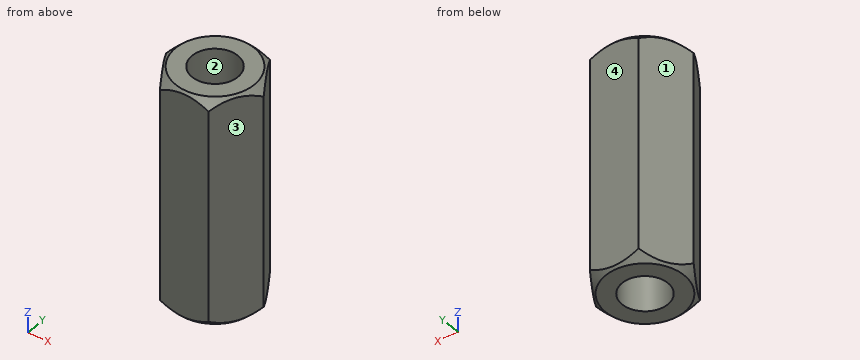
```python
from build123d import *

# Parameters (mm, degrees)
EXTRUDE_1_DEPTH   = 4
HOLE_WIZARD_M21_D = 1.6


with BuildPart() as part:
    # Эскиз1 → Бобышка-Вытянуть1 (new, symmetric)
    with BuildSketch(Plane.XY):
        Polygon((1.674315781, 0), (0.83715789, 1.45), (-0.83715789, 1.45), (-1.674315781, 0), (-0.83715789, -1.45), (0.83715789, -1.45), align=None)
    extrude(amount=EXTRUDE_1_DEPTH, both=True)

    # Отверстие обработанное метчиком M21 (through all)
    with Locations(Plane.XY.offset(4)):
        with Locations((0, 0)):
            Hole(HOLE_WIZARD_M21_D / 2)

    # Эскиз4 → Вырез-Повернуть1 (revolve, cut)
    with BuildSketch(Plane(origin=(0, 0, 0), x_dir=(0, 0, -1), z_dir=(0, 1, 0)), mode=Mode.PRIVATE) as cut_revolve_1_sk:
        Polygon((4, 1.374315781), (3.7, 1.674315781), (4, 1.674315781), align=None)
        Polygon((-4, 1.674315781), (-4, 1.374315781), (-3.7, 1.674315781), align=None)
    revolve(cut_revolve_1_sk.sketch.rotate(Axis((0, 0, -4), (0, 0, 1)), 180), axis=Axis((0, 0, -4), (0, 0, 1)), mode=Mode.SUBTRACT)


solid = part.part
```
Geometry check sheet. Reference: the model listing, model coordinates, mm. Face numbers are marked on the shaded views. Round coordinates to 2 decimals unless told otherwise and drop trailing zeros. Loops run counter-clockwise (first coordinate to the right, second up) from the corner with the lowest first, then second, coordinate; pieces in that order, holes last. Notation, with made-up numbers: (-20.5, 48) -> (35.5, 48) arc R24 cw to (35.5, 67) -> close; hole circle Ø9 at (27, 6). An arc over 180 degrees is marked (long way). Use a Markdown table: item, result.
(1) Scan lines: probe 1 along Y at (x, z) = (0, -1.25); probe 2 along X at (y, z) = (-0.4, 0); probe 3 along X at (y, z) = (-0.1, -3.25). Record each from-to range of solid material in increasing order.
Calculated:
| item | result |
|---|---|
| probe 1 | -1.45 to -0.8, 0.8 to 1.45 |
| probe 2 | -1.44 to -0.69, 0.69 to 1.44 |
| probe 3 | -1.62 to -0.79, 0.79 to 1.62 |
(2) Sectioned sample at B-B (z = -0.75). Enter the section's corners in (x, y), then the cut area to 3 significant figures.
Calculated:
| item | result |
|---|---|
| outline | (-1.67, 0) -> (-0.84, -1.45) -> (0.84, -1.45) -> (1.67, 0) -> (0.84, 1.45) -> (-0.84, 1.45) -> close; hole circle Ø1.6 at (0, 0) |
| area | 5.27 mm² |
(3) Go/stop test with flat-tipped pins: P1, Ø1.5, axis at y = -0.5, z = 2.5, coming from the -X side; P2, Ø1.4, axis at x = 0, y = 0, coming from the -Z side. Record where each tip stops, or that it passes through.
Calculated:
| item | result |
|---|---|
| P1 | x = -1.67 |
| P2 | through |
(4) Mould release check, pull along X, two halves, no side actions. Record for the marked faces 1, 2, 3 and 4: released by +X, released by -X, zero draft, split by the parting line, or undercut.
Calculated:
| item | result |
|---|---|
| face 1 | released by -X |
| face 2 | undercut |
| face 3 | released by +X |
| face 4 | zero draft |
(5) Sectioned sample at A-A (x = 0). Enter the section's corners in (y, z).
Calculated:
| item | result |
|---|---|
| outline | (-1.45, -3.92) -> (-1.37, -4) -> (-0.8, -4) -> (-0.8, 4) -> (-1.37, 4) -> (-1.45, 3.92) -> close; (0.8, -4) -> (1.37, -4) -> (1.45, -3.92) -> (1.45, 3.92) -> (1.37, 4) -> (0.8, 4) -> close |
